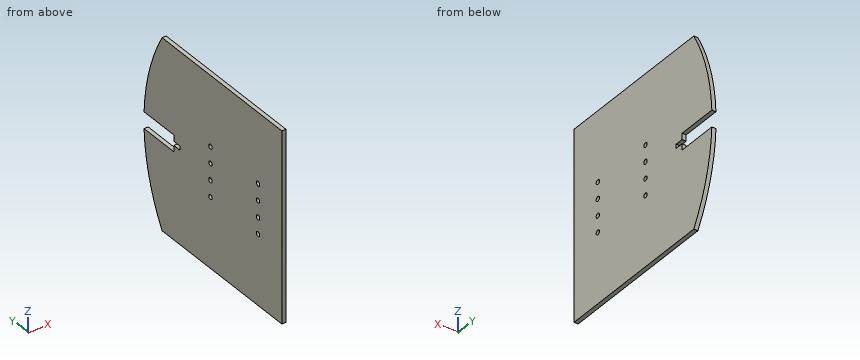
from build123d import *

# Parameters (mm, degrees)
BOSS_EXTRUDE1_DEPTH = 6.35
SKETCH2_R           = 3.5687
CUT_EXTRUDE1_DEPTH  = 149.606


with BuildPart() as part:
    # Sketch1 → Boss-Extrude1 (new body)
    with BuildSketch(Plane(origin=(0, 0, 0), x_dir=(0, 0, -1), z_dir=(1, 0, 0))):
        with BuildLine():
            Line((0, 0), (146.05, 0))
            Line((146.05, 0), (146.05, 255.602258394))
            ThreePointArc((146.05, 255.602258394), (81.677042764, 282.828530529), (12.7, 294.111929367))
            Line((12.7, 294.111929367), (12.7, 230.611929367))
            Line((12.7, 230.611929367), (3.175, 230.611929367))
            Line((3.175, 230.611929367), (3.175, 217.911929367))
            Line((3.175, 217.911929367), (-3.175, 217.911929367))
            Line((-3.175, 217.911929367), (-3.175, 230.611929367))
            Line((-3.175, 230.611929367), (-12.7, 230.611929367))
            Line((-12.7, 230.611929367), (-12.7, 294.111929367))
            ThreePointArc((-12.7, 294.111929367), (-81.677042764, 282.828530529), (-146.05, 255.602258394))
            Line((-146.05, 255.602258394), (-146.05, 0))
            Line((-146.05, 0), (0, 0))
        make_face()
    extrude(amount=BOSS_EXTRUDE1_DEPTH)

    # Sketch2 → Cut-Extrude1 (cut)
    with BuildSketch(Plane(origin=(0, 0, 0), x_dir=(0, 0, -1), z_dir=(1, 0, 0))):
        with Locations(Location((12.7, 50.8, 0), (0, 0, 180))):
            Circle(SKETCH2_R)
        with Locations(Location((38.1, 50.8, 0), (0, 0, 180))):
            Circle(SKETCH2_R)
        with Locations(Location((12.7, 152.4, 0), (0, 0, 180))):
            Circle(SKETCH2_R)
        with Locations(Location((38.1, 152.4, 0), (0, 0, 180))):
            Circle(SKETCH2_R)
        with Locations(Location((-12.7, 50.8, 0), (0, 0, 180))):
            Circle(SKETCH2_R)
        with Locations(Location((-38.1, 50.8, 0), (0, 0, 180))):
            Circle(SKETCH2_R)
        with Locations(Location((-38.1, 152.4, 0), (0, 0, 180))):
            Circle(SKETCH2_R)
        with Locations(Location((-12.7, 152.4, 0), (0, 0, 180))):
            Circle(SKETCH2_R)
    extrude(amount=CUT_EXTRUDE1_DEPTH, mode=Mode.SUBTRACT)


solid = part.part
Check sheet for the modelled part. Datum: model origin and axes. Units: mm. Round coordinates to 2 decimals unless told otherwise and drop trailing zeros. Loops run counter-clockwise (first coordinate to the right, second up) from the corner with the lowest first, then second, coordinate; pieces in that order, holes last. Notation, with made-up numbers: (86, 6) - (123, 6) arc R24 cw to (123, 32) - close; hole circle Ø7 at (68.25, -39.5). An arc over 180 degrees is marked (long way). Answer as CSV lines item,"result". Start each with the question number.
Item 1: Section check B-B (x = 4.5). Count the separate pieces of the cut face and the enclosed holes in it, and give its area (3 significant figures).
Item 2: Scan lines: line 1 (Z direction, x = 3.5, y = 152.4); line 2 (Y direction, x = 4.75, z = -38.1); line 3 (Z direction, x = 2.5, y = 259). Record each from-to range of solid material in increasing order. Write a range as [from, to].
Item 3: Section check C-C (y = 226). Record the boundary of the cut face in (x, z) (3 decimals), and give its area (3 significant figures).
Item 4: Section check D-D (z = -38.1). Record the boundary of the cut face in (x, y).
Item 5: Depth check by flat-ended pin: P1, Ø6.5, axis at y = 50.8, z = 38.1, coming from the -X side; P2, Ø1.5, axis at x = 4, z = -94, coming from the +Y side; P3, Ø3, axis at x = 2, z = -8.5, coming from the +Y side. Enter the tip coordinate at first touch or a pass-through.
Item 6: Section check A-A (y = 152.4). Record the boundary of the cut face in (x, z), and give its area (3 significant figures).
Report:
1,separate pieces,"1"
1,enclosed holes,"8"
1,area,"80,300 mm2"
2,line 1,"z = [-146.05, -41.67], [-34.53, -16.27], [-9.13, 9.13], [16.27, 34.53], [41.67, 146.05]"
2,line 2,"y = [0, 47.23], [54.37, 148.83], [155.97, 291.91]"
2,line 3,"z = [-139.94, -12.7], [12.7, 139.94]"
3,outline,"(0, -146.05) - (6.35, -146.05) - (6.35, -3.175) - (0, -3.175) - close; (0, 3.175) - (6.35, 3.175) - (6.35, 146.05) - (0, 146.05) - close"
3,area,"1,810 mm2"
4,outline,"(0, 0) - (6.35, 0) - (6.35, 47.23) - (0, 47.23) - close; (0, 54.37) - (6.35, 54.37) - (6.35, 148.83) - (0, 148.83) - close; (0, 155.97) - (6.35, 155.97) - (6.35, 291.91) - (0, 291.91) - close"
5,P1,"passes through"
5,P2,"stops at y = 279.23"
5,P3,"stops at y = 230.61"
6,outline,"(0, -146.05) - (6.35, -146.05) - (6.35, -41.67) - (0, -41.67) - close; (0, -34.53) - (6.35, -34.53) - (6.35, -16.27) - (0, -16.27) - close; (0, -9.13) - (6.35, -9.13) - (6.35, 9.13) - (0, 9.13) - close; (0, 16.27) - (6.35, 16.27) - (6.35, 34.53) - (0, 34.53) - close; (0, 41.67) - (6.35, 41.67) - (6.35, 146.05) - (0, 146.05) - close"
6,area,"1,670 mm2"
